from build123d import *

# Parameters (mm, degrees)
F0_R     = 7.5
F1_DEPTH = 2
F2_R     = 6
F3_DEPTH = 5
F4_T     = -2


with BuildPart() as f1:
    # F0 (on Top) → F1 (new body)
    with BuildSketch(Plane.XY):
        Circle(F0_R)
    extrude(amount=F1_DEPTH)

    # F2 (on face) → F3 (join)
    with BuildSketch(Plane.XY.offset(2)):
        Circle(F2_R)
    extrude(amount=F3_DEPTH)

    # F4
    f4_openings = [f1.faces().sort_by_distance(p)[0] for p in [
        (0, 0, 7),
    ]]
    offset(amount=F4_T, openings=f4_openings, kind=Kind.INTERSECTION)


solid = f1.part
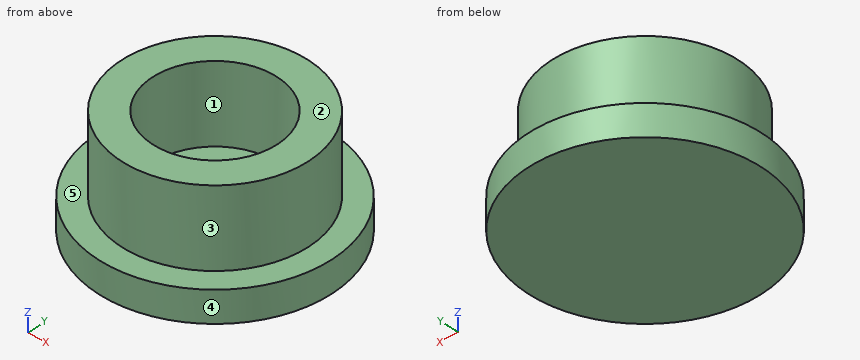
CAD build for the part. Positions are in the model's coordinates, mm. Face numbers are marked on the shaded views. A direction names the side the tool comes from. Coordinates: 2 decimals unless noted, no trailing zeros. Write each loop counter-clockwise with the first axis right and the second up, starting at its lowest first coordinate (ties: lowest second). Pieces come first, ordered by that corner, then holes. Notation, with made-up numbers: M 44,-22.75 L 57,-22.75 A14 cw 57,-17.75 Z; hole C 45,-8 d3. An arc over 180 degrees is marked long. Answer as a JSON object with one key per item and string values. Group by question number.
1) Saw through at C-C (z = 5.25). Write the cut outline in (x, y), plus the area to 3 significant figures.
2) Saw through at D-D (z = 0.5). Write the cut outline in (x, y), plus the area to 3 significant figures.
3) Saw through at A-A (y = 0). Write the cut outline in (x, z).
4) Saw through at B-B (x = 2.75). Write the cut outline in (y, z), plus the area to 3 significant figures.
5) Wall check: line 1 (Y direction, x = 0, z = 5.3); line 2 (Z direction, x = 0, y = -2.75); line 3 (Y direction, x = -3.5, z = 6.75). Give the ranges that are in metal, low to high. Write a range as from..to.
6) Mould opens along Y. For the marked faces 1, 2 and 3 say: +Y half, -Y half, draft (parallel to the pull), parting line (faces both ways), or undercut.
7) Pin check, flat tips, straight feed: pin 1 Ø4 at (y, z) = (1.5, 1.5) entering from -X; pin 2 Ø1 at (y, z) = (0.5, 6) entering from -X; pin 3 Ø1.5 at (y, z) = (2, 4.5) entering from +X; pin 4 Ø2 at (x, z) = (2, 6) entering from -Y. Stop position of each tip, or through.
8) Tool access for the marked faces 4 and 5: list every direction of +Z, -Z, +X, -X, +Y, -Y with a clear straight run to the whole face (end or side of a thin tool).
Values follow:
{
 "1": {"outline": "C 0,0 d12; hole C 0,0 d8", "area": "62.8 mm2"},
 "2": {"outline": "C 0,0 d15", "area": "177 mm2"},
 "3": {"outline": "M -7.5,0 L 7.5,0 L 7.5,2 L 6,2 L 6,7 L 4,7 L 4,2 L -4,2 L -4,7 L -6,7 L -6,2 L -7.5,2 Z"},
 "4": {"outline": "M -6.98,0 L 6.98,0 L 6.98,2 L 5.33,2 L 5.33,7 L 2.9,7 L 2.9,2 L -2.9,2 L -2.9,7 L -5.33,7 L -5.33,2 L -6.98,2 Z", "area": "52.2 mm2"},
 "5": {"line 1": "y = -6..-4, 4..6", "line 2": "z = 0..2", "line 3": "y = -4.87..-1.94, 1.94..4.87"},
 "6": {"face 1": "undercut", "face 2": "draft", "face 3": "parting line"},
 "7": {"pin 1": "stops at x = -7.5", "pin 2": "stops at x = -6", "pin 3": "stops at x = 5.87", "pin 4": "stops at y = -5.92"},
 "8": {"face 4": "+Z, -Z", "face 5": "+Z"}
}
